Autodesk Inventor part; units mm, degrees
ref_plane "YZ Plane" through (0, 0, 0) normal (1, 0, 0) x (0, 1, 0)
ref_plane "XZ Plane" through (0, 0, 0) normal (0, 1, 0) x (-1, 0, 0)
ref_plane "XY Plane" through (0, 0, 0) normal (0, 0, 1) x (1, 0, 0)
sketch "Sketch1" plane through (0, 0, 0) normal (0, 1, 0) x (-1, 0, 0)
  line L0 (10, -6.5) -> (-30, -6.5)
  line L1 (10, -10.5) -> (14, -10.5)
  line L2 (14, -10.5) -> (14, 0)
  line L3 (10, -6.5) -> (10, -10.5)
  line L4 (-30, 0) -> (-30, -6.5)
  line L5 (10, 6.5) -> (-30, 6.5)
  line L6 (10, 10.5) -> (14, 10.5)
  line L7 (14, 10.5) -> (14, 0)
  line L8 (10, 6.5) -> (10, 10.5)
  line L9 (-30, 0) -> (-30, 6.5)
  point P0 (0, 0)
  dimension "d0" = 40
  dimension "d5" = 4
  dimension "d15" = 13
extrude "Extrusion1" add sketch "Sketch1" along normal blind 5
sketch "Sketch2" plane through (0, 5, 0) normal (0, 1, 0) x (1, 0, 0)
  circle A0 centre (25, 0) radius 2
  arc A1 (9, -2) -> (9, 2) centre (9, 0) ccw
  arc A2 (4.1943, 2) -> (4.1943, -2) centre (4.1943, 0) ccw
  line L0 (9, -2) -> (4.1943, -2)
  line L1 (4.1943, 2) -> (9, 2)
  point P0 (0, 0)
  dimension "d8" = 4
  dimension "d10" = 4
  dimension "d11" = 12
  dimension "d12" = 4
extrude "Extrusion2" cut sketch "Sketch2" against normal blind 7.75
properties part number "motor_fastening"
Source: CAD feature listing. Evaluate the final solid. Frame: model axes, mm. A direction names the side the tool comes from. Give positions to 0.01 mm unless a question says otherwise; leave off trailing zeros. Write each loop counter-clockwise with the first axis right and the second up, starting at its lowest first coordinate (ties: lowest second). Pieces come first, ordered by that corner, then holes. Notation, with made-up numbers: M -37,62 L -22,62 A23 cw -22,82 Z; hole C 53.5,-26.5 d9. An arc over 180 degrees is marked long. Return JSON: item names as keys, results as strings. Group by question number.
1) Pin query (flat end, axial travel): P1, Ø2, axis at x = 13, y = 2, coming from the +Z side; P2, Ø2, axis at y = 2, z = -9, coming from the +X side. Return the tip coordinate at first contact, or that it passes through.
2) Material intervals for line 1 along X through (y, z) = (2.85, 0); line 2 along Z through (x, y) = (25, 2.5); line 3 along Z through (x, y) = (17, 1.4), sorted ascending. Write a range as [from, to].
3) Set-up query: faces 1 (the face through (-10, 2, 8)), 2 (the face through (2.195, 2.535, -0.044)), 3 (the face through (8.3, 5, -2.2)), 4 (the face through (10, 2, -6.5)). Return all of +Z, -Z, +X, -X, +Y, -Y with unobstructed straight access to the full face (end or side cutting, diameter ignored); none if empty.
4) Cut plane A-A, the plane x = 8. Output: boundary loops of the cut face in (y, z).
5) Cut plane B-B, the plane z = 0. Output: boundary loops of the cut face in (x, y), plus the area to 3 significant figures.
6) Cut plane D-D, the plane z = 9. Output: boundary loops of the cut face in (x, y).
7) Pull-direction query (X, two-part tool) for faces 5 (the face through (10, 2, 6.5)), 6 (the face through (7, 3, -2)), 7 (the face through (-14, 2, 0)), 8 (the face through (-10, 2, -8)); classes: pulls with the +X half, pulls with the -X half, needs draft (parallel to the pull), parting line crosses it, or undercut.
8) Cut plane C-C, the plane y = 0.6. Output: boundary loops of the cut face in (x, z), plus the area to 3 significant figures.
Recorded:
{
 "1": {"P1": "stops at z = 6.5", "P2": "stops at x = -10"},
 "2": {"line 1": "x = [-14, 2.19], [11, 23], [27, 30]", "line 2": "z = [-6.5, -2], [2, 6.5]", "line 3": "z = [-6.5, 6.5]"},
 "3": {"face 1": "+Z, +X, +Y, -Y", "face 2": "+Y, -Y", "face 3": "+Z, -Z, +X, -X, +Y", "face 4": "-Z, +X, +Y, -Y"},
 "4": {"outline": "M 0,-6.5 L 5,-6.5 L 5,-2 L 0,-2 Z; M 0,2 L 5,2 L 5,6.5 L 0,6.5 Z"},
 "5": {"outline": "M -14,0 L 2.19,0 L 2.19,5 L -14,5 Z; M 11,0 L 23,0 L 23,5 L 11,5 Z; M 27,0 L 30,0 L 30,5 L 27,5 Z", "area": "156 mm²"},
 "6": {"outline": "M -14,0 L -10,0 L -10,5 L -14,5 Z"},
 "7": {"face 5": "needs draft", "face 6": "undercut", "face 7": "pulls with the -X half", "face 8": "pulls with the +X half"},
 "8": {"outline": "M -14,-10.5 L -10,-10.5 L -10,-6.5 L 30,-6.5 L 30,6.5 L -10,6.5 L -10,10.5 L -14,10.5 Z; hole M 4.19,-2 L 9,-2 A2 ccw 9,2 L 4.19,2 A2 ccw Z; hole C 25,0 d4", "area": "560 mm²"}
}
